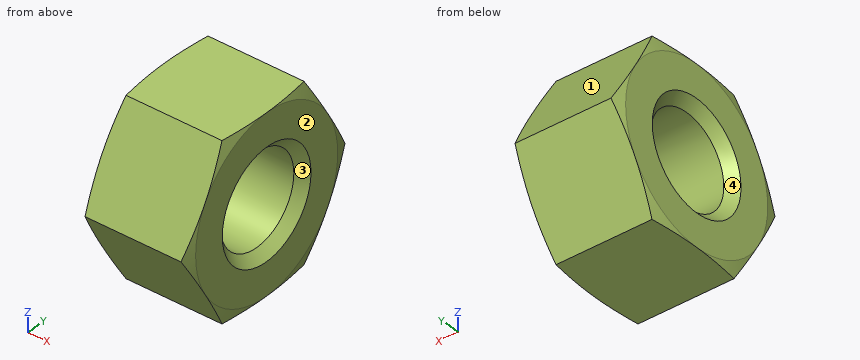
```python
from build123d import *

# Parameters (mm, degrees)
SKETCH3_W               = 16
SKETCH3_H               = 16
CUT_EXTRUDE1_DEPTH      = 4.7
CUT_EXTRUDE1_DEPTH_BACK = 4.7


with BuildPart() as part:
    # Sketch1 → Revolve1 (revolve)
    with BuildSketch(Plane.XY):
        Polygon((-2.35, 0), (-2.35, 4), (-2.135640646, 4.8), (2.135640646, 4.8), (2.35, 4), (2.35, 0), align=None)
    revolve(axis=Axis((2.35, 0, 0), (-1, 0, 0)))

    # Sketch2 → Cut-Revolve1 (revolve, cut)
    with BuildSketch(Plane.XY):
        Polygon((-2.35, 0), (-2.35, 2.5), (-1.917, 2.067), (1.917, 2.067), (2.35, 2.5), (2.35, 0), align=None)
    revolve(axis=Axis((2.35, 0, 0), (-1, 0, 0)), mode=Mode.SUBTRACT)

    # Sketch3 → Cut-Extrude1 (cut, two sides)
    with BuildSketch(Plane(origin=(0, 0, 0), x_dir=(0, 0, -1), z_dir=(1, 0, 0))) as cut_extrude1_sk:
        Rectangle(SKETCH3_W, SKETCH3_H)
        Polygon((-4, 2.309401077), (-4, -2.309401077), (0, -4.618802154), (4, -2.309401077), (4, 2.309401077), (0, 4.618802154), align=None, mode=Mode.SUBTRACT)
    extrude(amount=CUT_EXTRUDE1_DEPTH, mode=Mode.SUBTRACT)
    extrude(cut_extrude1_sk.sketch, amount=-CUT_EXTRUDE1_DEPTH_BACK, mode=Mode.SUBTRACT)


solid = part.part
```
Model file for the job. Use its own axes, mm. Face numbers are marked on the shaded views. Give positions to 0.01 mm unless a question says otherwise; leave off trailing zeros. Write each loop counter-clockwise with the first axis right and the second up, starting at its lowest first coordinate (ties: lowest second). Pieces come first, ordered by that corner, then holes. Notation, with made-up numbers: (84, 77) -> (105, 77) arc R26 cw to (105, 95) -> close; hole circle Ø5 at (44, -24.5). An arc over 180 degrees is marked (long way). Use CSV: the item, a comma, the result in double quotes. Start each with the question number.
1) Two-plate mould, pull along Z, no slides. Class the marked faces 1, 2, 3 and 4: released by +Z, released by -Z, zero draft, split by the parting line, or undercut.
2) Pin check, flat tip, straight feed: P1, Ø2, axis at y = 0, z = 0, coming from the +X side. Stop position of the tip, or through.
3) Cut at A-A on x = -1.6. List the corners of the cut face in (y, z).
4) Drill centre lines: L1, parallel to Y at x = 2.2, z = 1.25; L2, parallel to Y at x = -1.5, z = -0.5; L3, parallel to Z at x = 1.25, y = -0.75. Where is each one in solid material? Low to high.
Final values:
1,face 1,"released by +Z"
1,face 2,"zero draft"
1,face 3,"undercut"
1,face 4,"undercut"
2,P1,"passes through"
3,outline,"(-4.62, 0) -> (-2.31, -4) -> (2.31, -4) -> (4.62, 0) -> (2.31, 4) -> (-2.31, 4) -> close; hole circle Ø4.13 at (0, 0)"
4,L1,"y = -3.9 to -1.99, 1.99 to 3.9"
4,L2,"y = -4.33 to -2.01, 2.01 to 4.33"
4,L3,"z = -4 to -1.93, 1.93 to 4"
